Here's how the part is built. I have some questions about the finished solid (model axes, mm). Coordinates: 2 decimals unless noted, no trailing zeros. Write each loop counter-clockwise with the first axis right and the second up, starting at its lowest first coordinate (ties: lowest second). Pieces come first, ordered by that corner, then holes. Notation, with made-up numbers: (-39.75, 83) -> (0.25, 83) arc R10 ccw to (0.25, 91) -> close; hole circle Ø4 at (86, 73.25). An arc over 180 degrees is marked (long way). Answer in a Markdown table with one row per item. Add a question column.
from build123d import *


with BuildPart() as part:
    # Esquisse1 → Révolution1 (revolve)
    with BuildSketch(Plane.XY):
        with BuildLine():
            Line((0, 3.3), (0, 4.25))
            Line((0, 4.25), (0.95, 4.25))
            Line((0.95, 4.25), (27.5, 4.25))
            Line((27.5, 4.25), (28.318139594, 3.329592957))
            ThreePointArc((28.318139594, 3.329592957), (29.647828221, 2.26910367), (31.256068325, 1.715684176))
            Line((31.256068325, 1.715684176), (39.831964715, 0.327205713))
            ThreePointArc((39.831964715, 0.327205713), (39.952303879, 0.259405019), (40, 0.129776594))
            Line((40, 0.129776594), (40, 0))
            Line((40, 0), (30.006720572, 0))
            Line((30.006720572, 0), (27.073387239, 3.3))
            Line((27.073387239, 3.3), (0, 3.3))
        make_face()
    revolve(axis=Axis((0, 0, 0), (1, 0, 0)))


solid = part.part
Q1. I'm going to push flat-ended pins straight in: P1, Ø1.5, axis at x = 6, z = -1.5, coming from the -Y side; P2, Ø2, axis at x = 21, z = -2.5, coming from the -Y side. Where does each tip first touch, or does it pass through?
Q2. Imagine slicing it at A-A on x = 12. Please give me the cut outline in (y, z).
Q3. I need wall thicknesses on line 1 (Z direction, x = 19.75, y = 0); line 2 (Y direction, x = 8, z = -2.25); line 3 (Y direction, x = 11, z = 1.5). Which ranges of each line are inside material? Lowest first, please. Write a range as [from, to].
Q4. If we mould it in two halves opening along Z, with no side actions, what happens to faces 1 (the cylindrical face through (13.35, -2.43, 2.23)), 2 (the flat face through (0, -2, -3)), 3 (the conical face through (35.6, -0.75, 0.68))? For each: pulls with the +Z half, pulls with the -Z half, needs draft (parallel to the pull), parting line crosses it, or undercut.
Result sheet:
| question | item | result |
|---|---|---|
| 1 | P1 | stops at y = -4.18 |
| 1 | P2 | stops at y = -3.98 |
| 2 | outline | circle Ø8.5 at (0, 0); hole circle Ø6.6 at (0, 0) |
| 3 | line 1 | z = [-4.25, -3.3], [3.3, 4.25] |
| 3 | line 2 | y = [-3.61, -2.41], [2.41, 3.61] |
| 3 | line 3 | y = [-3.98, -2.94], [2.94, 3.98] |
| 4 | face 1 | undercut |
| 4 | face 2 | needs draft |
| 4 | face 3 | parting line crosses it |
